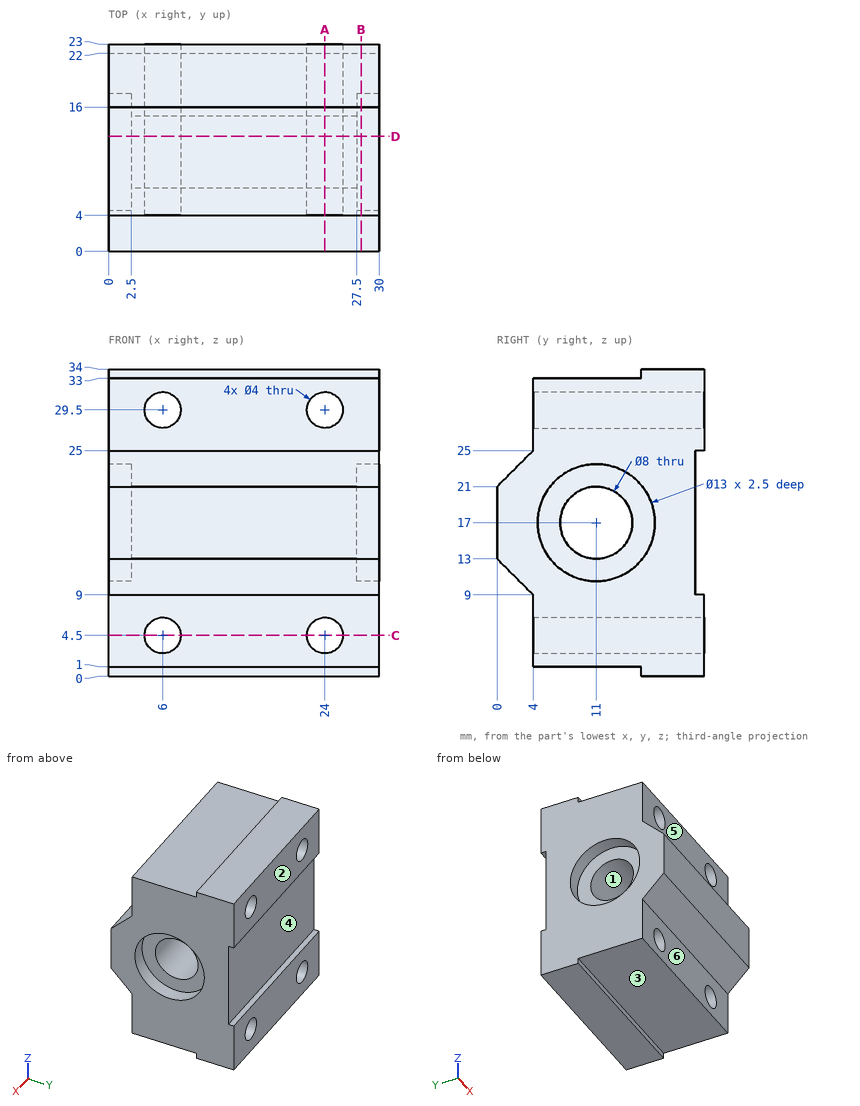
Geometry check sheet. Reference: drawing and pictorial views, mm from the part's lowest x, y, z. A direction names the side the tool comes from. Give positions to 0.01 mm unless a question says otherwise; leave off trailing zeros. Loops run counter-clockwise (first coordinate to the right, second up) from the corner with the lowest first, then second, coordinate; pieces in that order, holes last. Notation, with made-up numbers: (-28, 5.5) - (-23, 5.5) arc R29 ccw to (-23, 27.5) - close; hole circle Ø4 at (55, -29.75). An arc over 180 degrees is marked (long way). One line per question, with ' | ' between items. Start each with the question number.
1. Cross-section at D-D, the plane y = 12.75. Enter the section's corners in (x, z), plus the area to 3 significant figures.
2. Set-up check for the marked faces 4, 5 and 6: record each of +Z, -Z, +X, -X, +Y, -Y from which the full face is reachable in a straight line by a thin tool's end or side.
3. Cross-section at C-C, the plane z = 4.5. Enter the section's corners in (x, y).
4. Material ranges on line 1 along X through (y, z) = (13.5, 4.5); line 2 along Z through (x, y) = (15.5, 11); line 3 along Z through (x, y) = (24, 11.75), recorded low to high. Write a range as [from, to].
5. Cross-section at B-B, the plane x = 28. Enter the section's corners in (y, z).
6. Draft check along Z on the marked faces 1, 2 and 3. Enter one of: released by +Z, released by -Z, zero draft, split by the parting line, or undercut.
7. Cross-section at A-A, the plane x = 24. Enter the section's corners in (y, z).
8. Gauge pin test, flat ends, axial feed: pin 1 Ø2.5 at (x, z) = (24, 4.5) entering from -Y; pin 2 Ø8 at (x, z) = (6, 20.5) entering from -Y; pin 3 Ø6.5 at (x, z) = (9.5, 29) entering from -Y; pin 4 Ø3 at (x, y) = (24, 11) entering from -Z. Record the tip position at first contact, or that the pin passes through.
Check result:
1) outline: (0, 1) - (30, 1) - (30, 10.74) - (27.5, 10.74) - (27.5, 13.4) - (2.5, 13.4) - (2.5, 10.74) - (0, 10.74) - close; (0, 23.26) - (2.5, 23.26) - (2.5, 20.6) - (27.5, 20.6) - (27.5, 23.26) - (30, 23.26) - (30, 33) - (0, 33) - close; hole circle Ø4 at (6, 4.5); hole circle Ø4 at (6, 29.5); hole circle Ø4 at (24, 4.5); hole circle Ø4 at (24, 29.5) | area: 667 mm2
2) face 4: +X, -X, +Y | face 5: +Z, +X, -X, -Y | face 6: -Z, +X, -X, -Y
3) outline: (0, 4) - (4, 4) - (4, 23) - (0, 23) - close; (8, 4) - (22, 4) - (22, 23) - (8, 23) - close; (26, 4) - (30, 4) - (30, 23) - (26, 23) - close
4) line 1: x = [0, 4], [8, 22], [26, 30] | line 2: z = [1, 13], [21, 33] | line 3: z = [1, 2.5], [6.5, 13.07], [20.93, 27.5], [31.5, 33]
5) outline: (0, 13) - (4, 9) - (4, 1) - (16, 1) - (16, 0) - (23, 0) - (23, 9) - (22, 9) - (22, 25) - (23, 25) - (23, 34) - (16, 34) - (16, 33) - (4, 33) - (4, 25) - (0, 21) - close; hole circle Ø13 at (11, 17)
6) face 1: undercut | face 2: zero draft | face 3: released by -Z
7) outline: (0, 13) - (4, 9) - (4, 6.5) - (23, 6.5) - (23, 9) - (22, 9) - (22, 25) - (23, 25) - (23, 27.5) - (4, 27.5) - (4, 25) - (0, 21) - close; (4, 1) - (16, 1) - (16, 0) - (23, 0) - (23, 2.5) - (4, 2.5) - close; (4, 31.5) - (23, 31.5) - (23, 34) - (16, 34) - (16, 33) - (4, 33) - close; hole circle Ø8 at (11, 17)
8) pin 1: passes through | pin 2: stops at y = 0 | pin 3: stops at y = 4 | pin 4: stops at z = 1
